Answer from the drawing. Dimensions are ordinates in mm from the lowest x, y and z of the part. Give positions to 0.01 mm unless a question says otherwise; leave off trailing zeros. Write each loop counter-clockwise with the first axis right and the second up, starting at its lowest first coordinate (ties: lowest second). Pieces come first, ordered by that corner, then holes. Notation, with made-up numbers: (4.25, -19) -> (40.25, -19) arc R11 ccw to (40.25, -11) -> close; hole circle Ø9 at (80.25, 0.5). An arc over 180 degrees is marked (long way). Use a Markdown table: item, result. Add a question column.
Q1. Section B-B, the plane x = 258 is taken. Give the vertices of the cut face in (y, z).
Q2. Consider line 1 (X direction, y = 42.5, z = 2.9) (1 decimal); line 2 (X direction, y = 18.5, z = 0.9); line 3 (Y direction, x = 396, z = 0.3). Determine where each line is inside the solid, lowest interval first.
Q3. For a pull along Z with two mould halves and no side action, classify the marked faces 1 and 2 as pulls with the +Z half, pulls with the -Z half, needs draft (parallel to the pull), parting line crosses it, or undercut.
Q4. Section A-A, the plane z = 4.9 is taken. Give the vertices of the cut face in (x, y) (1 decimal), plus the area to 3 significant figures.
Q5. Section C-C, the plane y = 18 is taken. Give the vertices of the cut face in (x, z).
Q6. Each of these flat-tipped pins is pushed along its axis until it touches: pin 1 Ø3 at (y, z) = (21.5, 3) entering from -X; pin 2 Ø1.8 at (x, z) = (101.5, 2) entering from +Y. Where does it stop, or does it pass through?
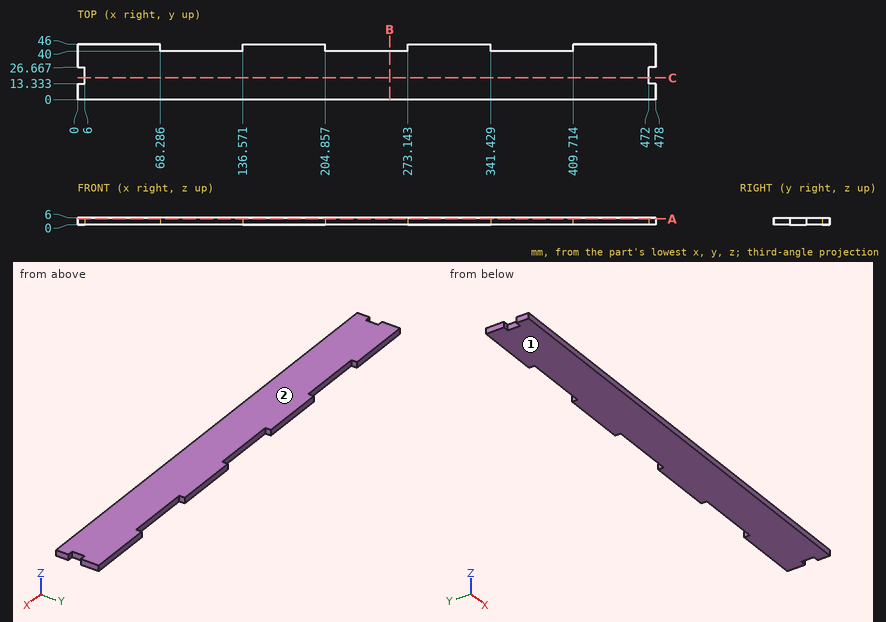
Result set:
| question | item | result |
|---|---|---|
| 1 | outline | (0, 0) -> (40, 0) -> (40, 6) -> (0, 6) -> close |
| 2 | line 1 | x = 0 to 68.3, 136.6 to 204.9, 273.1 to 341.4, 409.7 to 478 |
| 2 | line 2 | x = 6 to 472 |
| 2 | line 3 | y = 0 to 40 |
| 3 | face 1 | pulls with the -Z half |
| 3 | face 2 | pulls with the +Z half |
| 4 | outline | (0, 0) -> (478, 0) -> (478, 13.3) -> (472, 13.3) -> (472, 26.7) -> (478, 26.7) -> (478, 46) -> (409.7, 46) -> (409.7, 40) -> (341.4, 40) -> (341.4, 46) -> (273.1, 46) -> (273.1, 40) -> (204.9, 40) -> (204.9, 46) -> (136.6, 46) -> (136.6, 40) -> (68.3, 40) -> (68.3, 46) -> (0, 46) -> (0, 26.7) -> (6, 26.7) -> (6, 13.3) -> (0, 13.3) -> close |
| 4 | area | 20,600 mm2 |
| 5 | outline | (6, 0) -> (472, 0) -> (472, 6) -> (6, 6) -> close |
| 6 | pin 1 | stops at x = 6 |
| 6 | pin 2 | stops at y = 40 |
